Geometry: see drawing. Coordinates: mm, zero at the bounding-box minimum. Coordinates: 2 decimals unless noted, no trailing zeros. Write each loop counter-clockwise with the first axis right and the second up, starting at its lowest first coordinate (ties: lowest second). Pieces come first, ordered by that corner, then holes.
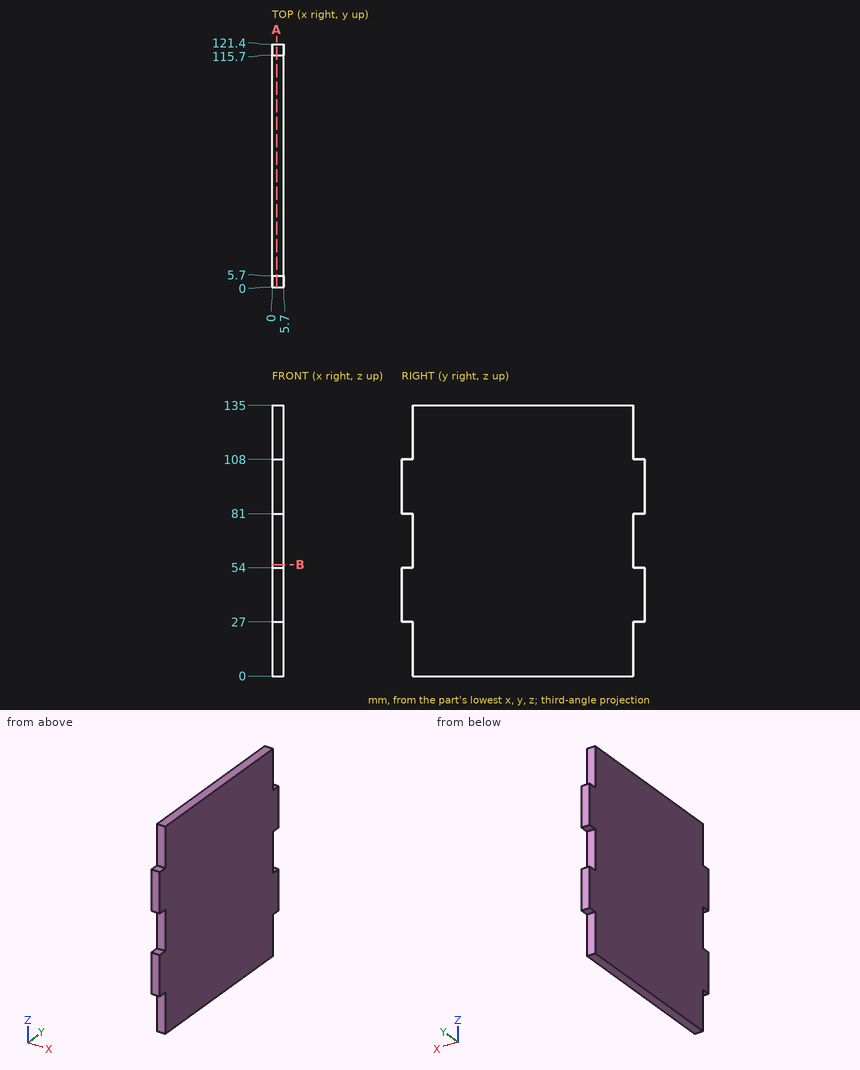
Item 1: Section B-B, the plane z = 55.5. Output: boundary loops of the cut face in (x, y), plus the area to 3 significant figures.
Derived:
outline: (0, 5.7) - (5.7, 5.7) - (5.7, 115.7) - (0, 115.7) - close
area: 627 mm2
Item 2: Pin query (flat end, axial travel): pin 1 (3 mm diameter, centred on x = 1.5, y = 120, fed in from +Z); pin 2 (2 mm diameter, centred on x = 3.5, z = 22.5, fed in from -Y); pin 3 (2 mm diameter, centred on x = 3, z = 61, fed in from +Y). Return the tip coordinate at first contact, or that it passes through.
Derived:
pin 1: stops at z = 108
pin 2: stops at y = 5.7
pin 3: stops at y = 115.7
Item 3: Material intervals for probe 1 along Y at (x, z) = (4.1, 114), sorted ascending.
Derived:
probe 1: y = 5.7 to 115.7
Item 4: Section A-A, the plane x = 2.3. Output: boundary loops of the cut face in (y, z).
Derived:
outline: (0, 27) - (5.7, 27) - (5.7, 0) - (115.7, 0) - (115.7, 27) - (121.4, 27) - (121.4, 54) - (115.7, 54) - (115.7, 81) - (121.4, 81) - (121.4, 108) - (115.7, 108) - (115.7, 135) - (5.7, 135) - (5.7, 108) - (0, 108) - (0, 81) - (5.7, 81) - (5.7, 54) - (0, 54) - close
